Autodesk Inventor part; units mm, degrees
ref_plane "YZ Plane" through (0, 0, 0) normal (1, 0, 0) x (0, 1, 0)
ref_plane "XZ Plane" through (0, 0, 0) normal (0, 1, 0) x (-1, 0, 0)
ref_plane "XY Plane" through (0, 0, 0) normal (0, 0, 1) x (1, 0, 0)
sketch "スケッチ1" plane through (0, 0, 0) normal (0, 0, 1) x (1, 0, 0)
  line L0 (7.5, 7.5) -> (-7.5, 7.5)
  line L1 (-7.5, 7.5) -> (-7.5, -7.5)
  line L2 (-7.5, -7.5) -> (7.5, -7.5)
  line L3 (7.5, -7.5) -> (7.5, 7.5)
  line L4 (7.5, 7.5) -> (-7.5, -7.5) construction
  line L5 (-7.5, 7.5) -> (7.5, -7.5) construction
  line L6 (-6, 6) -> (6, 6)
  line L7 (6, 6) -> (6, -6)
  line L8 (6, -6) -> (-6, -6)
  line L9 (-6, -6) -> (-6, 6)
  point P0 (0, 0)
  dimension "d0" = 15
  dimension "d1" = 15
  dimension "d2" = 1.5
extrude "押し出し1" add sketch "スケッチ1" along normal blind 552
sketch "スケッチ2" plane through (-7.5, 7.5, 0) normal (0, 1, 0) x (1, 0, 0)
  circle A0 centre (7.5, -7.5) radius 1.6
  line L0 (15, 0) -> (0, 0)
  circle A1 centre (7.5, -544.5) radius 1.6
  line L1 (15, -552) -> (0, -552)
  point P0 (7.5, 0)
  point P1 (7.5, 0)
  point P2 (7.5, -552)
  dimension "d5" = 3.2
  dimension "d6" = 7.5
  dimension "d7" = 3.2
  dimension "d8" = 7.5
extrude "押し出し2" cut sketch "スケッチ2" against normal through all
properties part number "上下機構_角柱5" material "アルミニウム 6061"
The listing builds one solid part. Answer for the finished solid, in the listing's coordinates (mm). A direction names the side the tool comes from. Round coordinates to 2 decimals unless told otherwise and drop trailing zeros. Order: outer loops, then holes, each group sorted by start corner. A loop starts at its lowest first (then second) coordinate and runs counter-clockwise, first axis right, second up. Notation, with made-up numbers: (56, 3.25) - (76, 3.25) arc R25 ccw to (76, 25.25) - close; hole circle Ø7 at (49, 11.25). An arc over 180 degrees is marked (long way). Write item = value, one per line. Start each with the question number.
1) For faces 4 (the flat face through (-6, 0, 272)), 5 (the flat face through (-7.5, 0, 272)), determine the directions among +Z, -Z, +X, -X, +Y, -Y from which every point of the face is accessible in a straight line to the end or side of a thin tool.
2) Section B-B, the plane z = 257.5 is taken. Write down the section's boundary in (x, y).
3) Straight lines are drawn through the part: L1, parallel to Z at x = 0, y = 6.4; L2, parallel to Y at x = 2.25, z = 432. For each, find the intervals that lie inside material, in ascending order.
4) For a pull along Z with two mould halves and no side action, classify faces 1 (the flat face through (7.5, 0, 272)), 2 (the flat face through (-7, 0, 552)), 3 (the flat face through (-7, 0, 0)) as released by +Z, released by -Z, zero draft, split by the parting line, or undercut.
5) Section A-A, the plane y = 1 is taken. Write down the section's boundary in (x, z).
Results list:
q1.face_4 = +Z, -Z
q1.face_5 = +Z, -Z, -X, +Y, -Y
q2.outline = (-7.5, -7.5) - (7.5, -7.5) - (7.5, 7.5) - (-7.5, 7.5) - close; hole (-6, -6) - (6, -6) - (6, 6) - (-6, 6) - close
q3.L1 = 0 to 5.9, 9.1 to 542.9, 546.1 to 552
q3.L2 = -7.5 to -6, 6 to 7.5
q4.face_1 = zero draft
q4.face_2 = released by +Z
q4.face_3 = released by -Z
q5.outline = (-7.5, 0) - (-6, 0) - (-6, 552) - (-7.5, 552) - close; (6, 0) - (7.5, 0) - (7.5, 552) - (6, 552) - close
